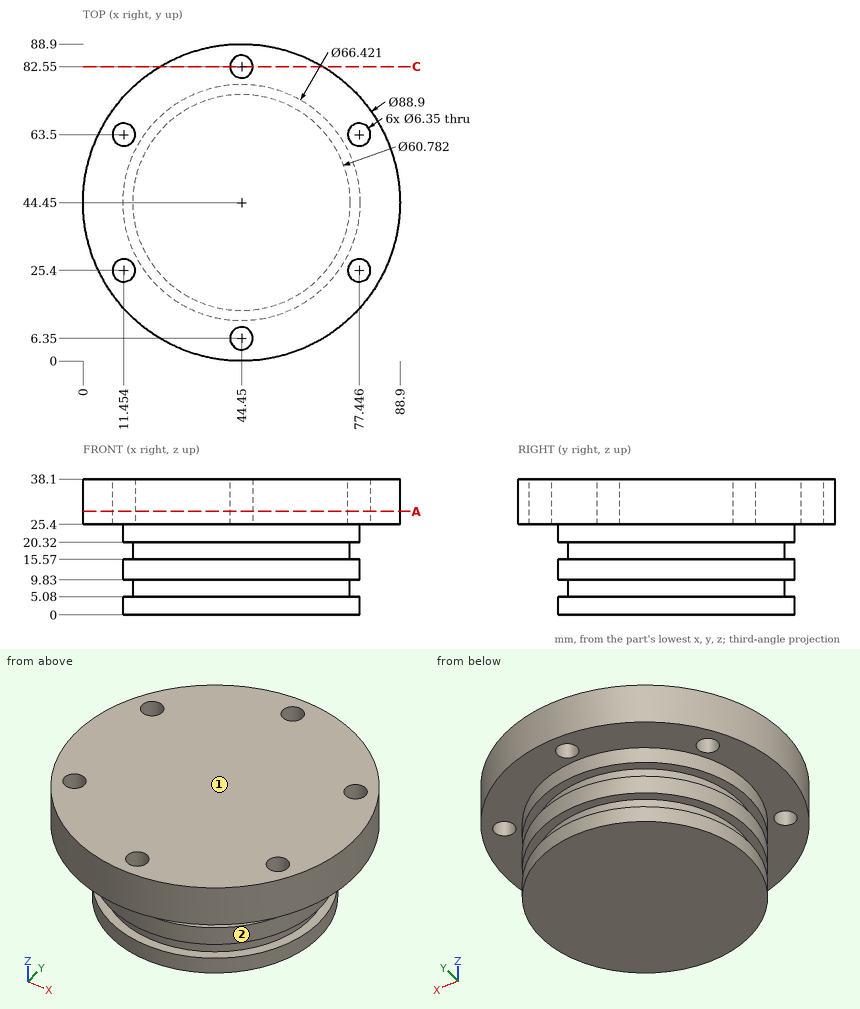
Input: dimensioned drawing with shaded views. Units: mm. Origin: part minimum x, y, z. A direction names the side the tool comes from. Give positions to 0.01 mm unless a question says otherwise; leave off trailing zeros. Write each loop counter-clockwise with the first axis right and the second up, starting at its lowest first coordinate (ties: lowest second). Pieces come first, ordered by that corner, then holes.
1. Material intervals for line 1 along Z through (x, y) = (28, 71); line 2 along X through (y, z) = (63, 33) (1 decimal); line 3 along X through (y, z) = (65, 35.5) (1 decimal), sorted ascending.
2. First-contact query: pin 1 (4 mm diameter, centred on x = 80, z = 7, fed in from +Y); pin 2 (5 mm diameter, centred on y = 13, z = 11, fed in from -X) (1 decimal); pin 3 (7.5 mm diameter, centred on x = 11.45, y = 63.5, fed in from -Z); pin 4 (4 mm diameter, centred on x = 27.5, z = 5.5, fed in from +Y). Flat tips, straight axial feed; report the tip coordinate or a pass-through.
3. Section query C-C (y = 82.55). Return the cut outline in (x, z) (1 decimal), then the cut area to 3 significant figures.
4. Access query for the marked faces 1 and 2. Directions: +Z, -Z, +X, -X, +Y, -Y. A direction counts if a zero-diameter tool reaches every point of the face in a straight line with its end or side. Return the directions, or none.
5. Section query A-A (z = 29). Count the separate pieces of the cut face and the enclosed holes in it, then the cut area to 3 significant figures.
Output values:
1. line 1: z = 0 to 5.08, 9.83 to 15.57, 20.32 to 38.1
1. line 2: x = 4.1 to 8.3, 14.6 to 74.3, 80.6 to 84.8
1. line 3: x = 5 to 8.7, 14.3 to 74.6, 80.2 to 83.9
2. pin 1: passes through
2. pin 2: stops at x = 28.2
2. pin 3: stops at z = 25.4
2. pin 4: stops at y = 74.08
3. outline: (21.6, 25.4) - (41.3, 25.4) - (41.3, 38.1) - (21.6, 38.1) - close; (47.6, 25.4) - (67.3, 25.4) - (67.3, 38.1) - (47.6, 38.1) - close
3. area: 501 mm2
4. face 1: +Z, +X, -X, +Y, -Y
4. face 2: -Z
5. separate pieces: 1
5. enclosed holes: 6
5. area: 6,020 mm2
